```python
from build123d import *

# Parameters (mm, degrees)
EXTRUDE_1_DEPTH     = 165
SKETCH_2_R          = 1.6
CUT_EXTRUDE_1_DEPTH = 284.20663834


with BuildPart() as part:
    # 草图1 → 凸台-拉伸1 (new body)
    with BuildSketch(Plane(origin=(0, 0, 0), x_dir=(1, 0, 0), z_dir=(0, 1, 0))):
        Polygon((0, 0), (83, 0), (83, -4), (230, -4), (230, -9), (83, -9), (0, -9), align=None)
    extrude(amount=EXTRUDE_1_DEPTH)

    # 草图2 → 切除-拉伸1 (cut, through all)
    with BuildSketch(Plane.XY.offset(9)):
        with Locations((227.5, 3)):
            Circle(SKETCH_2_R)
        with Locations((227.5, 155)):
            Circle(SKETCH_2_R)
        with Locations((80.5, 155)):
            Circle(SKETCH_2_R)
        with Locations((80.5, 3)):
            Circle(SKETCH_2_R)
        with Locations((2.5, 155)):
            Circle(SKETCH_2_R)
        with Locations((2.5, 3)):
            Circle(SKETCH_2_R)
    extrude(amount=-CUT_EXTRUDE_1_DEPTH, mode=Mode.SUBTRACT)


solid = part.part
```
Geometry: final body of the model. Coordinates: model frame, mm. A direction names the side the tool comes from. Round coordinates to 2 decimals unless told otherwise and drop trailing zeros. Order: outer loops, then holes, each group sorted by start corner. A loop starts at its lowest first (then second) coordinate and runs counter-clockwise, first axis right, second up. Notation, with made-up numbers: (16.5, 45.5) - (32.5, 45.5) arc R17 cw to (32.5, 61.5) - close; hole circle Ø6 at (-13, -9). An arc over 180 degrees is marked (long way). Write item = value, one per line. Start each with the question number.
Q1. Cut plane A-A on y = 16. Return the cut outline in (x, z), and give its area (3 significant figures).
Q2. Ray query, line 1 (Y direction, x = 227.5, z = 7.55); line 2 (X direction, y = 155, z = 5.2); line 3 (Z direction, x = 197, y = 137.5). Return the intervals inside material, ascending. Write a range as from..to.
Q3. Access query for faces 1 (the flat face through (155, 81, 4)), 2 (the flat face through (91, 165, 5)). Directions: +Z, -Z, +X, -X, +Y, -Y. A direction counts if a zero-diameter tool reaches every point of the face in a straight line with its end or side. Return the directions, or none.
Q4. Pin query (flat end, axial travel): pin 1 (1.5 mm diameter, centred on y = 52, z = 2.5, fed in from -X); pin 2 (3 mm diameter, centred on y = 115, z = 1.5, fed in from +X). Return the tip coordinate at first contact, or that it passes through.
Q5. Cut plane B-B on x = 175.5. Return the cut outline in (y, z), and give its area (3 significant figures).
Outcome:
q1.outline = (0, 0) - (83, 0) - (83, 4) - (230, 4) - (230, 9) - (0, 9) - close
q1.area = 1,480 mm^2
q2.line_1 = 0..1.4, 4.6..153.4, 156.6..165
q2.line_2 = 0..0.9, 4.1..78.9, 82.1..225.9, 229.1..230
q2.line_3 = 4..9
q3.face_1 = -Z, +X, +Y, -Y
q3.face_2 = +Z, -Z, +X, -X, +Y
q4.pin_1 = 0
q4.pin_2 = 83
q5.outline = (0, 4) - (165, 4) - (165, 9) - (0, 9) - close
q5.area = 825 mm^2
